Build history of the part. All positions in model axes, mm. Round coordinates to 2 decimals unless told otherwise and drop trailing zeros. Loops run counter-clockwise (first coordinate to the right, second up) from the corner with the lowest first, then second, coordinate; pieces in that order, holes last. Notation, with made-up numbers: (-2, 41) -> (53, 41) arc R22 ccw to (53, 54) -> close; hole circle Ø2 at (8.5, 82.5). An arc over 180 degrees is marked (long way). Put each result on its own line as item: value. Start each with the question number.
Item 1: Cut at A-A, the plane y = 0. Count the separate pieces of the cut face and the enclosed holes in it, plus the area to 3 significant figures.
Item 2: Drill centre lines: probe 1 along Z at (x, y) = (1.05, 0); probe 2 along Y at (x, z) = (1, -10.5); probe 3 along Z at (x, y) = (0.6, -1). Where is each one in solid material? Low to high. Write a range as [from, to].
Item 3: Cut at D-D, the plane z = -16.5. List the corners of the cut face in (x, y) (3 decimals), plus the area to 3 significant figures.
Item 4: Flat gauge pins, fed straight in: pin 1 Ø1 at (x, z) = (1, -63) entering from +Y; pin 2 Ø3 at (y, z) = (6.34, -9.86) entering from -X; pin 3 Ø1 at (x, z) = (1, -39) entering from +Y; pin 4 Ø1 at (x, z) = (2.5, -43.5) entering from -Y. Where does each tip first touch, or does it go through?
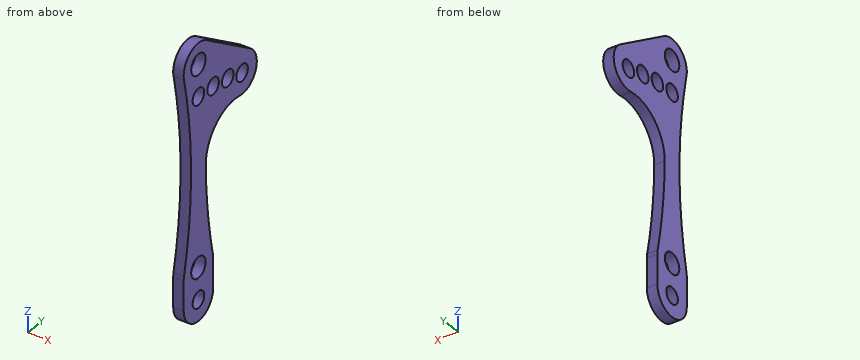
```python
from build123d import *

# Parameters (mm, degrees)
F0_R     = 2.4892
F0_R_2   = 3.1115
F1_DEPTH = 3.175


# Not quite as in the source:
# - ends of sketch curves that miss each other by under 0.0002 mm in the source are joined


with BuildPart() as f1:
    # F0 (on Right) → F1 (new body)
    with BuildSketch(Plane.YZ):
        with BuildLine():
            Line((22.3326001159, -7.2636385381), (3.5237049527, 5.2826133121))
            ThreePointArc((3.5237049527, 5.2826133121), (-3.5587166415, 5.2590907831), (-6.2140895311, -1.3067483686))
            ThreePointArc((-6.2140895311, -1.3067483686), (-3.1920426976, -30.3630411987), (-6.2140895148, -59.419334071))
            ThreePointArc((-6.2140895148, -59.419334071), (-6.3159309852, -60.0691839024), (-6.35, -60.7260825175))
            Line((-6.35, -60.7260825175), (-6.35, -69.5833))
            ThreePointArc((-6.35, -69.5833), (0, -75.9333), (6.35, -69.5833))
            Line((6.35, -69.5833), (6.35, -60.7259096378))
            ThreePointArc((6.35, -60.7259096378), (6.3159401222, -60.069098879), (6.2141258668, -59.419334071))
            ThreePointArc((6.2141258668, -59.419334071), (4.0014684949, -45.5311698082), (3.1652638563, -31.4927325362))
            ThreePointArc((3.1652638563, -31.4927325362), (7.4831947902, -21.8210036968), (17.6308936292, -18.7860284798))
            ThreePointArc((17.6308936292, -18.7860284798), (24.6882615086, -14.9453248745), (22.3326001159, -7.2636385381))
        make_face()
        with Locations((0, -69.5833)):
            Circle(F0_R, mode=Mode.SUBTRACT)
        with Locations((0, -60.0583)):
            Circle(F0_R_2, mode=Mode.SUBTRACT)
        with Locations((0, -9.525)):
            Circle(F0_R, mode=Mode.SUBTRACT)
        Circle(F0_R_2, mode=Mode.SUBTRACT)
        with Locations((6.3411204926, -9.86069465)):
            Circle(F0_R, mode=Mode.SUBTRACT)
        with Locations((12.6288141023, -10.8677786001)):
            Circle(F0_R, mode=Mode.SUBTRACT)
        with Locations((18.8088951631, -12.5462518503)):
            Circle(F0_R, mode=Mode.SUBTRACT)
    extrude(amount=F1_DEPTH)


solid = f1.part
```
Reply:
1. separate pieces: 5
1. enclosed holes: 0
1. area: 190 mm^2
2. probe 1: z = [-75.93, -72.07], [-67.09, -63.17], [-56.95, -12.01], [-7.04, -3.11], [3.11, 6.35]
2. probe 2: y = [-4.6, -2.29], [2.29, 3.94], [8.75, 10.17], [15.09, 17.39], [20.23, 24.82]
2. probe 3: z = [-75.85, -71.86], [-67.3, -63], [-57.11, -11.8], [-7.25, -2.95], [2.95, 6.27]
3. outline: (0, -3.874) -> (3.175, -3.874) -> (3.175, 23.778) -> (0, 23.778) -> close
3. area: 87.8 mm^2
4. pin 1: stops at y = 6.35
4. pin 2: passes through
4. pin 3: stops at y = 3.47
4. pin 4: stops at y = -3.85
